from build123d import *

# Parameters (mm, degrees)
F0_W          = 12.7
F0_H          = 1.016
F1_DEPTH      = 2.54
F1_DEPTH_BACK = 2.54
F0_W_2        = 25.4
F0_H_2        = 25.4
F2_DEPTH      = 2.54
F3_W          = 10.16
F3_H          = 1.016
F4_DEPTH      = 0.508
F4_TAPER      = 35


with BuildPart() as f1:
    # F0 (on Front) → F1 (new body, two sides)
    with BuildSketch(Plane.XZ) as f1_sk:
        with Locations((0, 8.89)):
            Rectangle(F0_W, F0_H)
    extrude(amount=F1_DEPTH)
    extrude(f1_sk.sketch, amount=-F1_DEPTH_BACK)

    # F0 (on Front) → F2 (join)
    with BuildSketch(Plane.XZ):
        Rectangle(F0_W_2, F0_H_2)
        with Locations((0, 8.89)):
            Rectangle(F0_W, F0_H, mode=Mode.SUBTRACT)
    extrude(amount=-F2_DEPTH)

    # F3 (on face) → F4 (join)
    with BuildSketch(Plane.XY.offset(9.398)):
        with Locations((0, -2.032)):
            Rectangle(F3_W, F3_H)
    extrude(amount=F4_DEPTH, taper=F4_TAPER)

    # F5: F1 across plane


with BuildPart() as f1_1:
    add(f1.part)
    add(f1.part.mirror(Plane.XY))


solid = f1_1.part
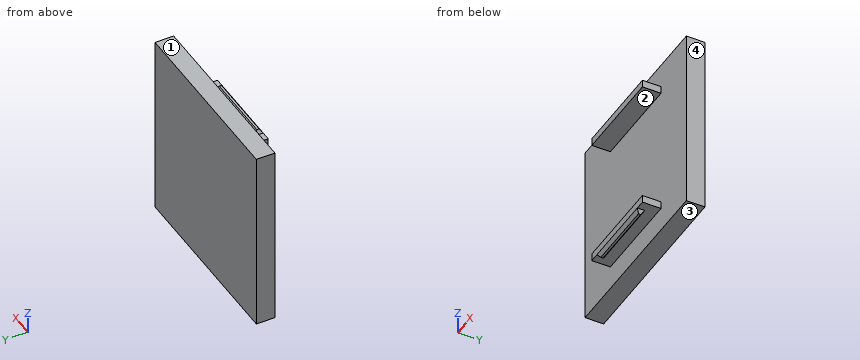
Check sheet for the modelled part. Datum: model origin and axes. Units: mm. Face numbers are marked on the shaded views. Give positions to 0.01 mm unless a question says otherwise; leave off trailing zeros. Loops run counter-clockwise (first coordinate to the right, second up) from the corner with the lowest first, then second, coordinate; pieces in that order, holes last. Notation, with made-up numbers: M 8.25,-17 L 48.25,-17 A28 ccw 48.25,19 Z; hole C -3.75,-10 d5. An arc over 180 degrees is marked long. Return JSON: item names as keys, results as strings. Group by question number.
1. Cross-section at D-D on x = 9.25. Record the boundary of the cut face in (y, z), plus the area to 3 significant figures.
2. Go/stop test with flat-tipped pins: pin 1 (3 mm diameter, centred on x = -1.5, y = -2, fed in from +Z); pin 2 (1.1 mm diameter, centred on y = -1, z = 9, fed in from +X); pin 3 (1.1 mm diameter, centred on y = -1, z = 8.5, fed in from -X); pin 4 (2 mm diameter, centred on y = -2, z = -3, fed in from +X). Record where each tip stops, or that it passes through.
3. Cross-section at A-A on y = -1.2. Record the boundary of the cut face in (x, z).
4. Mould release check, pull along Z, two halves, no side actions. Record for the marked faces 1, 2, 3 and 4: released by +Z, released by -Z, zero draft, split by the parting line, or undercut.
5. Cross-section at C-C on z = 4.25. Record the boundary of the cut face in (x, y), plus the area to 3 significant figures.
6. Cross-section at B-B on x = -1. Record the boundary of the cut face in (y, z), plus the area to 3 significant figures.
7. Thickness scan on L1, parallel to Z at x = 2.75, y = -0.5; L2, parallel to Y at x = 11.5, z = -7.5; L3, parallel to Y at x = -3.75, z = 9.5. Record the ranges inside material, lowest first.
Return value:
{
 "1": {"outline": "M 0,-12.7 L 2.54,-12.7 L 2.54,12.7 L 0,12.7 Z", "area": "64.5 mm^2"},
 "2": {"pin 1": "z = 9.91", "pin 2": "x = 6.35", "pin 3": "x = -6.35", "pin 4": "through"},
 "3": {"outline": "M -6.35,-9.4 L 6.35,-9.4 L 6.35,-8.38 L -6.35,-8.38 Z; M -6.35,8.38 L 6.35,8.38 L 6.35,9.4 L -6.35,9.4 Z"},
 "4": {"face 1": "released by +Z", "face 2": "undercut", "face 3": "released by -Z", "face 4": "zero draft"},
 "5": {"outline": "M -12.7,0 L 12.7,0 L 12.7,2.54 L -12.7,2.54 Z", "area": "64.5 mm^2"},
 "6": {"outline": "M -2.54,-9.4 L -2.18,-9.91 L -1.88,-9.91 L -1.52,-9.4 L 0,-9.4 L 0,-12.7 L 2.54,-12.7 L 2.54,12.7 L 0,12.7 L 0,9.4 L -1.52,9.4 L -1.88,9.91 L -2.18,9.91 L -2.54,9.4 L -2.54,8.38 L 0,8.38 L 0,-8.38 L -2.54,-8.38 Z", "area": "70.3 mm^2"},
 "7": {"L1": "-9.4 to -8.38, 8.38 to 9.4", "L2": "0 to 2.54", "L3": "-2.47 to -1.6, 0 to 2.54"}
}
